Here's how the part is built. I have some questions about the finished solid (model axes, mm). Coordinates: 2 decimals unless noted, no trailing zeros. Loops run counter-clockwise (first coordinate to the right, second up) from the corner with the lowest first, then second, coordinate; pieces in that order, holes last. Notation, with made-up numbers: (-4.75, 1) - (35.25, 1) arc R23 ccw to (35.25, 11) - close; hole circle Ø8 at (-13, -19). An arc over 180 degrees is marked (long way). Use a Markdown table: item, result.
```python
from build123d import *

# Parameters (mm, degrees)
F0_R     = 21.5
F1_DEPTH = 6


with BuildPart() as f1:
    # F0 (on Front) → F1 (new body)
    with BuildSketch(Plane.XZ):
        with BuildLine():
            Line((-43, -22.5), (-43, -25.5))
            Line((-43, -25.5), (43, -25.5))
            Line((43, -25.5), (43, -22.5))
            Line((43, -22.5), (25.5, 0))
            ThreePointArc((25.5, 0), (0, 25.5), (-25.5, 0))
            Line((-25.5, 0), (-43, -22.5))
        make_face()
        Circle(F0_R, mode=Mode.SUBTRACT)
    extrude(amount=F1_DEPTH)


solid = f1.part
```
Q1. If we mould it in two halves opening along X, with no side actions, what happens to faces 1 (the face through (0.561, -2.958, 25.494)), 2 (the face through (0, -6, -23)), 3 (the face through (-2.799, -2.958, 21.317)), 4 (the face through (34.372, -2.958, -11.407))? For each: pulls with the +X half, pulls with the -X half, needs draft (parallel to the pull), parting line crosses it, or undercut.
Check values:
| item | result |
|---|---|
| face 1 | parting line crosses it |
| face 2 | needs draft |
| face 3 | undercut |
| face 4 | pulls with the +X half |
Q2. Will this pin go through, and if not, where does the flat tip stop? P1, Ø2, axis at x = 1, y = -5, coming from the +Z side.
Check values:
| item | result |
|---|---|
| P1 | z = 25.5 |
Q3. I want a section at C-C, the plane y = -1.1. Write out the boundary of the cut face in (x, z), then the cut area to 3 significant figures.
Check values:
| item | result |
|---|---|
| outline | (-43, -25.5) - (43, -25.5) - (43, -22.5) - (25.5, 0) arc R25.5 ccw to (-25.5, 0) - (-43, -22.5) - close; hole circle Ø43 at (0, 0) |
| area | 1,370 mm^2 |
Q4. Please list where these lines run through material, in increasing order: L1, parallel to Z at x = 0, y = -3.4; L2, parallel to X at y = -1.75, z = 14.5; L3, parallel to X at y = -1.65, z = -8. Write a range as from..to.
Check values:
| item | result |
|---|---|
| L1 | -25.5..-21.5, 21.5..25.5 |
| L2 | -20.98..-15.87, 15.87..20.98 |
| L3 | -31.72..-19.96, 19.96..31.72 |
Q5. I want a section at A-A, the plane x = 0. Write out the boundary of the cut face in (y, z).
Check values:
| item | result |
|---|---|
| outline | (-6, -25.5) - (0, -25.5) - (0, -21.5) - (-6, -21.5) - close; (-6, 21.5) - (0, 21.5) - (0, 25.5) - (-6, 25.5) - close |
Q6. I want a section at D-D, the plane z = 22.5. Write out the boundary of the cut face in (x, y), then the cut area to 3 significant figures.
Check values:
| item | result |
|---|---|
| outline | (-12, -6) - (12, -6) - (12, 0) - (-12, 0) - close |
| area | 144 mm^2 |
Q7. I want a section at B-B, the plane z = -19.5. Write out the boundary of the cut face in (x, y), then the cut area to 3 significant figures.
Check values:
| item | result |
|---|---|
| outline | (-40.67, -6) - (-9.06, -6) - (-9.06, 0) - (-40.67, 0) - close; (9.06, -6) - (40.67, -6) - (40.67, 0) - (9.06, 0) - close |
| area | 379 mm^2 |
